Source: CAD feature listing. Evaluate the final solid. Frame: model axes, mm. Face numbers are marked on the shaded views. A direction names the side the tool comes from. Round coordinates to 2 decimals unless told otherwise and drop trailing zeros. Loops run counter-clockwise (first coordinate to the right, second up) from the corner with the lowest first, then second, coordinate; pieces in that order, holes last. Notation, with made-up numbers: (-20, -25.5) -> (-14, -25.5) arc R16 cw to (-14, 3.5) -> close; hole circle Ø7 at (-6, 44). An arc over 180 degrees is marked (long way). Put each result on its own line as item: value. Start each with the question number.
1. Set-up query: the marked faces 1 and 2. Return all of +Z, -Z, +X, -X, +Y, -Y with unobstructed straight access to the full face (end or side cutting, diameter ignored); none if empty.
2. Cut plane A-A (y = 4). Return the cut outline in (x, z), then the cut area to 3 significant figures.
3. Contact query for flat-ended pins moving along their axis: pin 1 (1.5 mm diameter, centred on x = 11.5, y = 0, fed in from +Z); pin 2 (13 mm diameter, centred on x = 0, y = 0, fed in from +Z); pin 3 (5 mm diameter, centred on x = 8.5, y = -11, fed in from +Z). Output: stop coordinate, or through.
4. Material intervals for L1, parallel to X at y = 0, z = 2.4; L2, parallel to Y at x = 11, z = 1.8; L3, parallel to Y at x = 9.75, z = 3.25, sorted ascending.
5. Draft query along X for the marked faces 3, 4 and 5. Return one class per face: pulls with the +X half, pulls with the -X half, needs draft (parallel to the pull), parting line crosses it, or undercut.
6. Cut plane C-C (z = 1.5). Return the cut outline in (x, y).
7. Cut plane D-D (y = 0). Return the cut outline in (x, z), then the cut area to 3 significant figures.
8. Cut plane B-B (x = 0). Return the cut outline in (y, z), then the cut area to 3 significant figures.
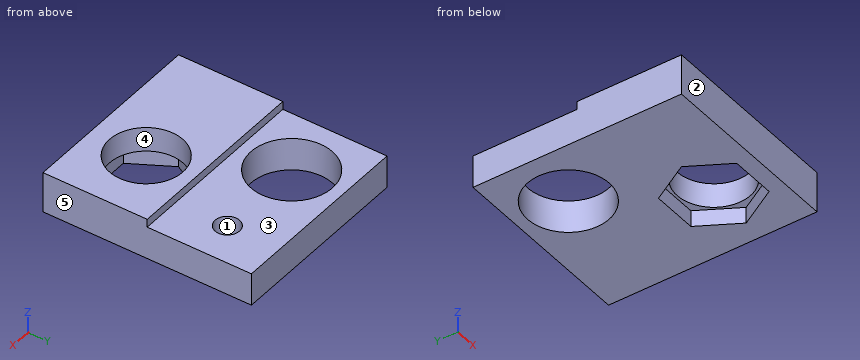
```python
from build123d import *

# Parameters (mm, degrees)
F0_W     = 23.179245647
F0_H     = 25.5798394792
F0_R     = 5
F0_R_2   = 1.5
F0_R_3   = 4.5
F1_DEPTH = 5
F2_DEPTH = 2
F3_START = 1
F3_DEPTH = 4
F4_W     = 23.179245647
F4_H     = 12.7899197396
F4_R     = 5
F4_R_2   = 1.5
F5_DEPTH = 1


with BuildPart() as f1:
    # F0 (on Top) → F1 (new body)
    with BuildSketch(Plane.XY):
        with Locations((4.2594347615, -6.3512411434)):
            Rectangle(F0_W, F0_H)
        Polygon((2.1032405912, -12.3641875159), (4.8745218833, -7.5641875159), (10.4170844675, -7.5641875159), (13.1883657596, -12.3641875159), (10.4170844675, -17.1641875159), (4.8745218833, -17.1641875159), align=None, mode=Mode.SUBTRACT)
        Circle(F0_R, mode=Mode.SUBTRACT)
        with Locations((11, 0)):
            Circle(F0_R_2, mode=Mode.SUBTRACT)
        Polygon((10.4170844675, -7.5641875159), (4.8745218833, -7.5641875159), (2.1032405912, -12.3641875159), (4.8745218833, -17.1641875159), (10.4170844675, -17.1641875159), (13.1883657596, -12.3641875159), align=None)
        with Locations((7.6458031754, -12.3641875159)):
            Circle(F0_R_3, mode=Mode.SUBTRACT)
        with Locations((11, 0)):
            Circle(F0_R_2)
    extrude(amount=F1_DEPTH)

    # F0 (on Top) → F2 (cut)
    with BuildSketch(Plane.XY):
        Polygon((10.4170844675, -7.5641875159), (4.8745218833, -7.5641875159), (2.1032405912, -12.3641875159), (4.8745218833, -17.1641875159), (10.4170844675, -17.1641875159), (13.1883657596, -12.3641875159), align=None)
        with Locations((7.6458031754, -12.3641875159)):
            Circle(F0_R_3, mode=Mode.SUBTRACT)
    extrude(amount=F2_DEPTH, mode=Mode.SUBTRACT)

    # F0 (on Top) → F3 (cut)
    with BuildSketch(Plane.XY.offset(F3_START)):
        with Locations((11, 0)):
            Circle(F0_R_2)
    extrude(amount=F3_DEPTH, mode=Mode.SUBTRACT)

    # F4 (on face) → F5 (cut)
    with BuildSketch(Plane.XY.offset(5)):
        with Locations((4.2594347615, 0.0437187264)):
            Rectangle(F4_W, F4_H)
        Circle(F4_R, mode=Mode.SUBTRACT)
        with Locations((11, 0)):
            Circle(F4_R_2, mode=Mode.SUBTRACT)
        with Locations((4.2594347615, 0.0437187264)):
            Rectangle(F4_W, F4_H)
    extrude(amount=-F5_DEPTH, mode=Mode.SUBTRACT)


solid = f1.part
```
Solution:
1. face 1: +Z
1. face 2: +Z, -Z, +X, -X, -Y
2. outline: (-7.33, 0) -> (-3, 0) -> (-3, 4) -> (-7.33, 4) -> close; (3, 0) -> (15.85, 0) -> (15.85, 4) -> (3, 4) -> close
2. area: 68.7 mm^2
3. pin 1: stops at z = 1
3. pin 2: stops at z = 5
3. pin 3: passes through
4. L1: x = -7.33 to -5, 5 to 9.5, 12.5 to 15.85
4. L2: y = -19.14 to -16.15, -8.57 to -1.5, 1.5 to 6.44
4. L3: y = -19.14 to -16.34, -8.39 to -0.83, 0.83 to 6.44
5. face 3: needs draft
5. face 4: undercut
5. face 5: pulls with the +X half
6. outline: (-7.33, -19.14) -> (15.85, -19.14) -> (15.85, 6.44) -> (-7.33, 6.44) -> close; hole circle Ø10 at (0, 0); hole (2.1, -12.36) -> (4.87, -17.16) -> (10.42, -17.16) -> (13.19, -12.36) -> (10.42, -7.56) -> (4.87, -7.56) -> close; hole circle Ø3 at (11, 0)
7. outline: (-7.33, 0) -> (-5, 0) -> (-5, 4) -> (-7.33, 4) -> close; (5, 0) -> (15.85, 0) -> (15.85, 4) -> (12.5, 4) -> (12.5, 1) -> (9.5, 1) -> (9.5, 4) -> (5, 4) -> close
7. area: 43.7 mm^2
8. outline: (-19.14, 0) -> (-5, 0) -> (-5, 4) -> (-6.35, 4) -> (-6.35, 5) -> (-19.14, 5) -> close; (5, 0) -> (6.44, 0) -> (6.44, 4) -> (5, 4) -> close
8. area: 75.1 mm^2
